Here's how the part is built. I have some questions about the finished solid (model axes, mm). Give positions to 0.01 mm unless a question says otherwise; leave off trailing zeros. Loops run counter-clockwise (first coordinate to the right, second up) from the corner with the lowest first, then second, coordinate; pieces in that order, holes last.
Q1. If we section it at A-A (y = 3.05): Please give me the cut outline in (x, z) (3 decimals).
Q2. I need wall thicknesses on line 1 (Y direction, x = 3.05, z = 1.8); line 2 (Y direction, x = 4.5, z = 0.5); line 3 (X direction, y = 3.25, z = 1.05). Which ranges of each line are inside material? Lowest first, please.
Q3. If we section it at C-C (z = 1.7): Please give me the cut outline in (x, y), plus the area to 3 significant figures.
Q4. We'd pull the mould along Y, two halves only. Please class faces 1 (the face through (0, 3, 1)), 2 (the face through (3, 0, 1)), 3 (the face through (5.48, 3.82, 1.51)): +Y half, -Y half, draft (parallel to the pull), parting line (faces both ways), or undercut.
from build123d import *

# Parameters (mm, degrees)
SKETCH1_W           = 6.1
SKETCH1_H           = 6.1
BOSS_EXTRUDE1_DEPTH = 2.975
CUT_EXTRUDE1_REACH  = 11.125
SKETCH2_R           = 2.55


with BuildPart() as part:
    # Sketch1 → Boss-Extrude1 (new body)
    with BuildSketch(Plane.XY):
        with Locations((3.05, 3.05)):
            Rectangle(SKETCH1_W, SKETCH1_H)
    extrude(amount=BOSS_EXTRUDE1_DEPTH)

    # Sketch2 → Cut-Extrude1 (cut, up to next)
    with BuildSketch(Plane.XY.offset(2.975), mode=Mode.PRIVATE) as cut_extrude1_sk1:
        with Locations((3.05, 3.05)):
            Circle(SKETCH2_R)
    cut_extrude1_tool1 = extrude(cut_extrude1_sk1.sketch, amount=-CUT_EXTRUDE1_REACH, mode=Mode.PRIVATE) & part.part
    add(cut_extrude1_tool1.solids().sort_by_distance((3.05, 3.05, 2.975))[0], mode=Mode.SUBTRACT)


solid = part.part
Check sheet entries:
1. outline: (0, 0) - (0.5, 0) - (0.5, 2.975) - (0, 2.975) - close; (5.6, 0) - (6.1, 0) - (6.1, 2.975) - (5.6, 2.975) - close
2. line 1: y = 0 to 0.5, 5.6 to 6.1
2. line 2: y = 0 to 0.95, 5.15 to 6.1
2. line 3: x = 0 to 0.51, 5.59 to 6.1
3. outline: (0, 0) - (6.1, 0) - (6.1, 6.1) - (0, 6.1) - close; hole circle Ø5.1 at (3.05, 3.05)
3. area: 16.8 mm2
4. face 1: draft
4. face 2: -Y half
4. face 3: undercut
